Design review of the part built by this model. Coordinates are the model's own, in mm. A direction names the side the tool comes from. Round coordinates to 2 decimals unless told otherwise and drop trailing zeros. Write each loop counter-clockwise with the first axis right and the second up, starting at its lowest first coordinate (ties: lowest second). Pieces come first, ordered by that corner, then holes.
from build123d import *

# Parameters (mm, degrees)
SKETCH_5_W          = 56
SKETCH_5_H          = 3
EXTRUDE_1_DEPTH     = 5
CUT_EXTRUDE_1_REACH = 58.303
SKETCH_6_R          = 1.6
CUT_EXTRUDE_2_REACH = 58.303
SKETCH_7_R          = 0.9
FILLET_1_R          = 1.5
SKETCH_8_W          = 6
SKETCH_8_H          = 1.6
CUT_EXTRUDE_3_DEPTH = 10
SKETCH_10_R         = 1.6
SKETCH_10_R_2       = 0.9
EXTRUDE_2_DEPTH     = 0.5
EXTRUDE_START       = 0.5
SKETCH_11_R         = 0.9
SKETCH_11_R_2       = 1.6
EXTRUDE_3_DEPTH     = 0.5
SKETCH_12_W         = 6.20639004
SKETCH_12_H         = 2
CUT_EXTRUDE_4_DEPTH = 10


with BuildPart() as part:
    # 草图5 → 凸台-拉伸1 (new body)
    with BuildSketch(Plane(origin=(0, 0, 0), x_dir=(1, 0, 0), z_dir=(0, 1, 0))):
        with Locations((28, -1.5)):
            Rectangle(SKETCH_5_W, SKETCH_5_H)
    extrude(amount=EXTRUDE_1_DEPTH)

    # 草图6 → 切除-拉伸1 (cut, up to next)
    with BuildSketch(Plane.XY.offset(3), mode=Mode.PRIVATE) as cut_extrude_1_sk1:
        with Locations((2.5, 2.5)):
            Circle(SKETCH_6_R)
    cut_extrude_1_tool1 = extrude(cut_extrude_1_sk1.sketch, amount=-CUT_EXTRUDE_1_REACH, mode=Mode.PRIVATE) & part.part
    add(cut_extrude_1_tool1.solids().sort_by_distance((2.5, 2.5, 3))[0], mode=Mode.SUBTRACT)

    # 草图7 → 切除-拉伸2 (cut, up to next)
    with BuildSketch(Plane.XY, mode=Mode.PRIVATE) as cut_extrude_2_sk1:
        with Locations(Location((54, 2.5, 0), (0, 0, 180))):
            Circle(SKETCH_7_R)
    cut_extrude_2_tool1 = extrude(cut_extrude_2_sk1.sketch, amount=CUT_EXTRUDE_2_REACH, mode=Mode.PRIVATE) & part.part
    add(cut_extrude_2_tool1.solids().sort_by_distance((54, 2.5, 0))[0], mode=Mode.SUBTRACT)

    # 圆角1
    fillet_1_edges = [part.edges().sort_by_distance(p)[0] for p in [
        (56, 5, 1.5),
        (56, 0, 1.5),
        (0, 0, 1.5),
        (0, 5, 1.5),
    ]]
    fillet(fillet_1_edges, radius=FILLET_1_R)

    # 草图8 → 切除-拉伸3 (cut)
    with BuildSketch(Plane(origin=(0, 5, 0), x_dir=(1, 0, 0), z_dir=(0, 1, 0))):
        with Locations((53, -1.5)):
            Rectangle(SKETCH_8_W, SKETCH_8_H)
    extrude(amount=-CUT_EXTRUDE_3_DEPTH, mode=Mode.SUBTRACT)

    # 草图10 → 凸台-拉伸2 (add)
    with BuildSketch(Plane.XY.offset(3)):
        with BuildLine():
            Line((56, 1.5), (56, 3.5))
            ThreePointArc((56, 3.5), (55.560660172, 4.560660172), (54.5, 5))
            Line((54.5, 5), (1.5, 5))
            ThreePointArc((1.5, 5), (0.439339828, 4.560660172), (0, 3.5))
            Line((0, 3.5), (0, 1.5))
            ThreePointArc((0, 1.5), (0.439339828, 0.439339828), (1.5, 0))
            Line((1.5, 0), (54.5, 0))
            ThreePointArc((54.5, 0), (55.560660172, 0.439339828), (56, 1.5))
        make_face()
        with Locations((2.5, 2.5)):
            Circle(SKETCH_10_R, mode=Mode.SUBTRACT)
        with Locations(Location((54, 2.5, 0), (0, 0, 180))):
            Circle(SKETCH_10_R_2, mode=Mode.SUBTRACT)
    extrude(amount=EXTRUDE_2_DEPTH)

    # 草图11 → 凸台-拉伸3 (add)
    with BuildSketch(Plane(origin=(0, 0, 0), x_dir=(-1, 0, 0), z_dir=(0, 0, -1)).offset(EXTRUDE_START)):
        with BuildLine():
            Line((-1.5, 5), (-54.5, 5))
            ThreePointArc((-54.5, 5), (-55.560660172, 4.560660172), (-56, 3.5))
            Line((-56, 3.5), (-56, 1.5))
            ThreePointArc((-56, 1.5), (-55.560660172, 0.439339828), (-54.5, 0))
            Line((-54.5, 0), (-1.5, 0))
            ThreePointArc((-1.5, 0), (-0.439339828, 0.439339828), (0, 1.5))
            Line((0, 1.5), (0, 3.5))
            ThreePointArc((0, 3.5), (-0.439339828, 4.560660172), (-1.5, 5))
        make_face()
        with Locations((-54, 2.5)):
            Circle(SKETCH_11_R, mode=Mode.SUBTRACT)
        with Locations(Location((-2.5, 2.5, 0), (0, 0, 180))):
            Circle(SKETCH_11_R_2, mode=Mode.SUBTRACT)
    extrude(amount=-EXTRUDE_3_DEPTH)

    # 草图12 → 切除-拉伸4 (cut)
    with BuildSketch(Plane(origin=(0, 5, 0), x_dir=(1, 0, 0), z_dir=(0, 1, 0))):
        with Locations((53.10319502, -1.5)):
            Rectangle(SKETCH_12_W, SKETCH_12_H)
    extrude(amount=-CUT_EXTRUDE_4_DEPTH, mode=Mode.SUBTRACT)


solid = part.part
1) For P1, Ø1.6, axis at y = 3, z = 1.5, coming from the +X side, flat-tipped, find the tip position at first contact; note if it passes through.
2) Add section C-C on z = 1.1. State the section outline as (x, y) points, and give its area (3 significant figures).
3) Add section D-D on x = 2.5. State the section outline as (y, z) points, and give its area (3 significant figures).
4) For faces 1 (the face through (50, 3, 2)), 2 (the face through (56, 2, 3)), list the 3-axis set-ups (+Z, -Z, +X, -X, +Y, -Y) from which the entire face can be reached by the end or side of a thin tool; tool diameter is ignored.
5) Add section A-A on x = 54. State the section outline as (y, z) points.
6) The part is to be moulded in two halves that separate along Z. For faces 3 (the face through (0.43, 4.55, 1.47)), 4 (the face through (28, 3, 3.5)), 5 (the face through (53, 3, 0.5)), say which applies: pulls with the +Z half, pulls with the -Z half, needs draft (parallel to the pull), parting line crosses it, or undercut.
7) For line 1 along X through (y, z) = (2.6, 0.3); line 2 along Y through (x, z) = (2.5, 3.45); line 3 along Z through (x, y) = (53.5, 4.45), list the stretches that pass through material, from the lowest coordinate up.
8) Add section B-B on y = 2.5. State the section outline as (x, z) points.
Computed:
1. P1: stops at x = 50
2. outline: (0, 1.5) arc R1.5 ccw to (1.5, 0) - (50, 0) - (50, 5) - (1.5, 5) arc R1.5 ccw to (0, 3.5) - close; hole circle Ø3.2 at (2.5, 2.5)
2. area: 241 mm2
3. outline: (0, -0.5) - (0.9, -0.5) - (0.9, 3.5) - (0, 3.5) - close; (4.1, -0.5) - (5, -0.5) - (5, 3.5) - (4.1, 3.5) - close
3. area: 7.20 mm2
4. face 1: +X, +Y, -Y
4. face 2: +Z, -Z, +X, +Y, -Y
5. outline: (0, -0.5) - (1.6, -0.5) - (1.6, 0.5) - (0, 0.5) - close; (0, 2.5) - (1.6, 2.5) - (1.6, 3.5) - (0, 3.5) - close; (3.4, -0.5) - (5, -0.5) - (5, 0.5) - (3.4, 0.5) - close; (3.4, 2.5) - (5, 2.5) - (5, 3.5) - (3.4, 3.5) - close
6. face 3: needs draft
6. face 4: pulls with the +Z half
6. face 5: undercut
7. line 1: x = 0 to 0.9, 4.1 to 53.11, 54.89 to 56
7. line 2: y = 0 to 0.9, 4.1 to 5
7. line 3: z = -0.5 to 0.5, 2.5 to 3.5
8. outline: (0, -0.5) - (0.9, -0.5) - (0.9, 3.5) - (0, 3.5) - close; (4.1, -0.5) - (53.1, -0.5) - (53.1, 0.5) - (50, 0.5) - (50, 2.5) - (53.1, 2.5) - (53.1, 3.5) - (4.1, 3.5) - close; (54.9, -0.5) - (56, -0.5) - (56, 0.5) - (54.9, 0.5) - close; (54.9, 2.5) - (56, 2.5) - (56, 3.5) - (54.9, 3.5) - close
